```python
from build123d import *

# Parameters (mm, degrees)
SKETCH1_W           = 155.575
SKETCH1_H           = 12.7
SKETCH1_W_2         = 12.7
SKETCH1_H_2         = 6.35
BOSS_EXTRUDE1_DEPTH = 25.4
SKETCH2_R           = 3.175
CUT_EXTRUDE1_DEPTH  = 13.7


with BuildPart() as part:
    # Sketch1 → Boss-Extrude1 (new body, symmetric)
    with BuildSketch(Plane.XY):
        Rectangle(SKETCH1_W, SKETCH1_H)
        with Locations((71.4375, 9.525)):
            Rectangle(SKETCH1_W_2, SKETCH1_H_2)
        with Locations((42.8625, 9.525)):
            Rectangle(SKETCH1_W_2, SKETCH1_H_2)
        with Locations((14.2875, 9.525)):
            Rectangle(SKETCH1_W_2, SKETCH1_H_2)
        with Locations((-14.2875, 9.525)):
            Rectangle(SKETCH1_W_2, SKETCH1_H_2)
        with Locations((-71.4375, 9.525)):
            Rectangle(SKETCH1_W_2, SKETCH1_H_2)
        with Locations((-42.8625, 9.525)):
            Rectangle(SKETCH1_W_2, SKETCH1_H_2)
    extrude(amount=BOSS_EXTRUDE1_DEPTH, both=True)

    # Sketch2 → Cut-Extrude1 (cut, through all)
    with BuildSketch(Plane(origin=(0, 6.35, 0), x_dir=(1, 0, 0), z_dir=(0, 1, 0))):
        Circle(SKETCH2_R)
        with Locations((-28.575, 0)):
            Circle(SKETCH2_R)
        with Locations((-57.15, 0)):
            Circle(SKETCH2_R)
    cut_extrude1 = extrude(amount=-CUT_EXTRUDE1_DEPTH, mode=Mode.SUBTRACT)

    # Mirror1: Cut-Extrude1 across plane
    add(cut_extrude1.mirror(Plane(origin=(0, 0, 0), x_dir=(0, 0, 1), z_dir=(1, 0, 0))), mode=Mode.SUBTRACT)


solid = part.part
```
Geometry check sheet. Reference: the model listing, model coordinates, mm. A direction names the side the tool comes from. Give positions to 0.01 mm unless a question says otherwise; leave off trailing zeros. Order: outer loops, then holes, each group sorted by start corner. A loop starts at its lowest first (then second) coordinate and runs counter-clockwise, first axis right, second up. Notation, with made-up numbers: (74, 75.25) - (106, 75.25) arc R22 ccw to (106, 109.25) - close; hole circle Ø6 at (73.5, -0.75). An arc over 180 degrees is marked (long way). Answer in a Markdown table with one row per item. Add a question column.
Q1. Mould release check, pull along X, two halves, no side actions. Record for faces 3 (the flat face through (77.788, 3, 0)), 4 (the flat face through (-1, 1, -25.4)), 5 (the flat face through (-20.638, 9, 0)): pulls with the +X half, pulls with the -X half, needs draft (parallel to the pull), parting line crosses it, or undercut.
Q2. Cross-section at B-B, the plane x = -57.15. Enter the section's corners in (y, z) (3 decimals).
Q3. Tool access check on faces 1 (the flat face through (43, 12.7, 0)), 2 (the flat face through (49.212, 9, 0)). Record the directions out of +Z, -Z, +X, -X, +Y, -Y that give a thin tool (end or side, any length) a straight path to the whole face; none if there is none.
Q4. Cross-section at C-C, the plane y = -0.5. Count the separate pieces of the cut face and the enclosed holes in it, then the cut area to 3 significant figures.
Q5. Material ranges on probe 1 along X at (y, z) = (9.5, -10); probe 2 along Z at (x, y) = (-29, 3); probe 3 along Z at (x, y) = (57.15, -0.75) (3 decimals), recorded low to high. Write a range as from..to.
Q6. Cross-section at D-D, the plane z = 17. Enter the section's corners in (x, y), then the cut area to 3 significant figures.
Q7. Cross-section at A-A, the plane y = 10. Enter the section's corners in (x, z), then the cut area to 3 significant figures.
Q8. Gauge pin test, flat end, axial feed: pin 1 (6 mm diameter, centred on x = -61, z = 20, fed in from +Y). Record the tip position at first contact, or that the pin passes through.
Check values:
| question | item | result |
|---|---|---|
| 1 | face 3 | pulls with the +X half |
| 1 | face 4 | needs draft |
| 1 | face 5 | undercut |
| 2 | outline | (-6.35, -25.4) - (6.35, -25.4) - (6.35, -3.175) - (-6.35, -3.175) - close; (-6.35, 3.175) - (6.35, 3.175) - (6.35, 25.4) - (-6.35, 25.4) - close |
| 3 | face 1 | +Z, -Z, +X, -X, +Y |
| 3 | face 2 | +Z, -Z, +Y |
| 4 | separate pieces | 1 |
| 4 | enclosed holes | 5 |
| 4 | area | 7,740 mm^2 |
| 5 | probe 1 | x = -77.79..-65.09, -49.21..-36.51, -20.64..-7.94, 7.94..20.64, 36.51..49.21, 65.09..77.79 |
| 5 | probe 2 | z = -25.4..-3.15, 3.15..25.4 |
| 5 | probe 3 | z = -25.4..-3.175, 3.175..25.4 |
| 6 | outline | (-77.79, -6.35) - (77.79, -6.35) - (77.79, 12.7) - (65.09, 12.7) - (65.09, 6.35) - (49.21, 6.35) - (49.21, 12.7) - (36.51, 12.7) - (36.51, 6.35) - (20.64, 6.35) - (20.64, 12.7) - (7.94, 12.7) - (7.94, 6.35) - (-7.94, 6.35) - (-7.94, 12.7) - (-20.64, 12.7) - (-20.64, 6.35) - (-36.51, 6.35) - (-36.51, 12.7) - (-49.21, 12.7) - (-49.21, 6.35) - (-65.09, 6.35) - (-65.09, 12.7) - (-77.79, 12.7) - close |
| 6 | area | 2,460 mm^2 |
| 7 | outline | (-77.79, -25.4) - (-65.09, -25.4) - (-65.09, 25.4) - (-77.79, 25.4) - close; (-49.21, -25.4) - (-36.51, -25.4) - (-36.51, 25.4) - (-49.21, 25.4) - close; (-20.64, -25.4) - (-7.94, -25.4) - (-7.94, 25.4) - (-20.64, 25.4) - close; (7.94, -25.4) - (20.64, -25.4) - (20.64, 25.4) - (7.94, 25.4) - close; (36.51, -25.4) - (49.21, -25.4) - (49.21, 25.4) - (36.51, 25.4) - close; (65.09, -25.4) - (77.79, -25.4) - (77.79, 25.4) - (65.09, 25.4) - close |
| 7 | area | 3,870 mm^2 |
| 8 | pin 1 | stops at y = 6.35 |
